```python
from build123d import *

# Parameters (mm, degrees)
F0_W      = 90.2540013194
F0_H      = 76.625905931
F1_DEPTH  = 75.184
F2_W      = 87.2799269855
F2_H      = 48.7919023726
F3_DEPTH  = 9.144
F4_W      = 48.7919023726
F4_H      = 9.144
F5_DEPTH  = 66.802
F6_W      = 48.7919023726
F6_H      = 9.144
F7_DEPTH  = 91.948
F8_W      = 90.2540013194
F8_H      = 12.7788623795
F9_DEPTH  = 8.636
F10_DEPTH = 55.372


with BuildPart() as f1:
    # F0 (on Front) → F1 (new body)
    with BuildSketch(Plane.XZ):
        with Locations((2.9570385814, -6.9426186383)):
            Rectangle(F0_W, F0_H)
    extrude(amount=F1_DEPTH)

    # F2 (on face) → F3 (join)
    with BuildSketch(Plane.XY.offset(31.3703343272)):
        with Locations((4.4440757483, -40.5677921372)):
            Rectangle(F2_W, F2_H)
    extrude(amount=F3_DEPTH)

    # F4 (on face) → F5 (join)
    with BuildSketch(Plane.YZ.offset(48.0840392411)):
        with Locations((-40.5677921372, 35.9423343272)):
            Rectangle(F4_W, F4_H)
    extrude(amount=F5_DEPTH)

    # F6 (on face) → F7 (join)
    with BuildSketch(Plane(origin=(-39.1958877444, 0, 0), x_dir=(0, -1, 0), z_dir=(-1, 0, 0))):
        with Locations((40.5677921372, 35.9423343272)):
            Rectangle(F6_W, F6_H)
    extrude(amount=F7_DEPTH)

    # F8 (on face) → F9 (join)
    with BuildSketch(Plane.XY.offset(31.3703343272)):
        Polygon((-132.288813591, 43.4794910252), (-132.288813591, -12.7788623795), (-42.1699620783, -12.7788623795), (-42.1699620783, 0), (48.0840392411, 0), (48.0840392411, -12.7788623795), (113.7418448925, -12.7788623795), (113.7418448925, 43.4794910252), align=None)
        with Locations((2.9570385814, -6.3894311897)):
            Rectangle(F8_W, F8_H)
    extrude(amount=F9_DEPTH)

    # F10 (add): a face of the model
    f10_faces = [f1.faces().sort_by_distance(p)[0] for p in [
        (2.9570385814, 0, -6.9426186383),
    ]]
    extrude(f10_faces, amount=F10_DEPTH)


solid = f1.part
```
Part model, mm, in its own coordinate system. A direction names the side the tool comes from. Give positions to 0.01 mm unless a question says otherwise; leave off trailing zeros. Write each loop counter-clockwise with the first axis right and the second up, starting at its lowest first coordinate (ties: lowest second). Pieces come first, ordered by that corner, then holes. Notation, with made-up numbers: M 8,-9 L 66,-9 A13 ccw 66,14 Z; hole C -28,40 d4. An arc over 180 degrees is marked long. Use CSV: the item, a comma, the result in double quotes.
Item 1: Slice it at C-C on x = -27.5. Write the cut outline in (y, z), plus the area to 3 significant figures.
Taken from the geometry:
outline,"M -75.18,-45.26 L 55.37,-45.26 L 55.37,31.37 L 43.48,31.37 L 43.48,40.01 L -12.78,40.01 L -12.78,31.37 L -16.17,31.37 L -16.17,40.51 L -64.96,40.51 L -64.96,31.37 L -75.18,31.37 Z"
area,"10,900 mm²"
Item 2: Pin check, flat tips, straight feed: P1, Ø2.5, axis at x = 7, z = 37, coming from the +Y side; P2, Ø17, axis at x = -84.5, y = 22, coming from the -Z side; P3, Ø23, axis at y = 22, z = -12, coming from the +X side; P4, Ø10, axis at x = 50.5, z = 35, coming from the -Y side. Stop position of each tip, or through.
Taken from the geometry:
P1,"stops at y = 43.48"
P2,"stops at z = 31.37"
P3,"stops at x = 48.08"
P4,"stops at y = -75.18"
Item 3: Pull direction Y, two halves, no side cores. Call faces 4 (the face through (-6, -64.964, 36)), 5 (the face through (2, 55.372, -6)), 6 (the face through (-11, -12.779, 36)), 7 (the face through (81, -41, 31.37)): +Y half, -Y half, draft (parallel to the pull), parting line (faces both ways), or undercut.
Taken from the geometry:
face 4,"-Y half"
face 5,"+Y half"
face 6,"undercut"
face 7,"draft"
Item 4: Slice it at A-A on x = -68. Write the cut outline in (y, z), plus the area to 3 significant figures.
Taken from the geometry:
outline,"M -64.96,31.37 L -16.17,31.37 L -16.17,40.51 L -64.96,40.51 Z; M -12.78,31.37 L 43.48,31.37 L 43.48,40.01 L -12.78,40.01 Z"
area,"932 mm²"
Item 5: Drill centre lines: probe 1 along Z at (x, y) = (-93, -22); probe 2 along Z at (x, y) = (68, 33); probe 3 along X at (y, z) = (-6, -6). Where is each one in solid material? Low to high.
Taken from the geometry:
probe 1,"z = 31.37 to 40.51"
probe 2,"z = 31.37 to 40.01"
probe 3,"x = -42.17 to 48.08"
Item 6: Which spindle directions (+Z, -Z, +X, -X, +Y, -Y) get a long thin tool onto all of the face, cutting with end or side? Do faces 1 (the face through (-11, 16, 40.006)), 2 (the face through (-86, -40, 31.37)), 3 (the face through (113.742, 15, 36)). Say none if no direction does.
Taken from the geometry:
face 1,"+Z, +X, -X, +Y"
face 2,"-Z, -X, +Y, -Y"
face 3,"+Z, -Z, +X, +Y"
Item 7: Slice it at D-D on z = 11. Write the cut outline in (x, y).
Taken from the geometry:
outline,"M -42.17,-75.18 L 48.08,-75.18 L 48.08,55.37 L -42.17,55.37 Z"
Item 8: Slice it at B-B on y = 1.5. Write the cut outline in (x, z), plus the area to 3 significant figures.
Taken from the geometry:
outline,"M -132.29,31.37 L -42.17,31.37 L -42.17,-45.26 L 48.08,-45.26 L 48.08,31.37 L 113.74,31.37 L 113.74,40.01 L -132.29,40.01 Z"
area,"9,040 mm²"
